Can you work these out from the model? Positions are in its coordinate system, mm. Face numbers are marked on the shaded views. A direction names the side the tool comes from. Round coordinates to 2 decimals unless told otherwise and drop trailing zeros. Order: outer loops, then holes, each group sorted by start corner. A loop starts at its lowest first (then second) coordinate and runs counter-clockwise, first axis right, second up. Notation, with made-up numbers: M 36,55 L 56,55 A26 ccw 56,75 Z; hole C -38.75,44 d2. An arc over 180 degrees is marked long. Answer as a JSON object with one key per item and string values. Group by question number.
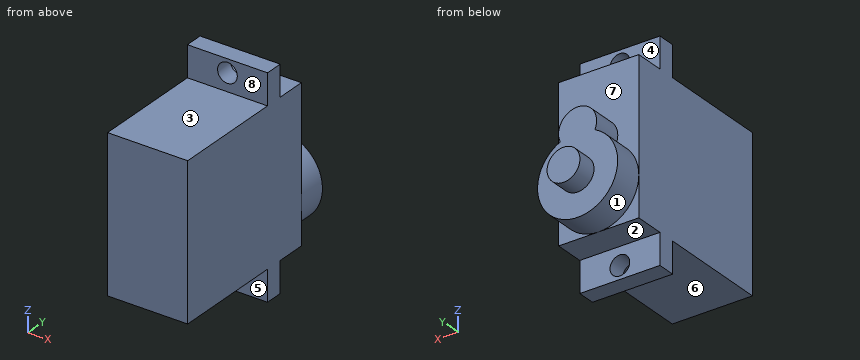
from build123d import *

# Parameters (mm, degrees)
SKETCH1_W           = 12.2
SKETCH1_H           = 23.2
BOSS_EXTRUDE3_DEPTH = 24.2
SKETCH5_W           = 12.2
SKETCH5_H           = 2.7
BOSS_EXTRUDE4_DEPTH = 4.7
CUT_EXTRUDE4_START  = -20.7
SKETCH6_R           = 1.5
CUT_EXTRUDE4_DEPTH  = 26.2
SKETCH7_R           = 2.9
SKETCH7_R_2         = 6.1
BOSS_EXTRUDE5_DEPTH = 4.5
SKETCH8_R           = 2.5
BOSS_EXTRUDE6_DEPTH = 3


with BuildPart() as part:
    # Sketch1 → Boss-Extrude3 (new body)
    with BuildSketch(Plane(origin=(0, 0, 0), x_dir=(1, 0, 0), z_dir=(0, 1, 0))):
        Rectangle(SKETCH1_W, SKETCH1_H)
    extrude(amount=BOSS_EXTRUDE3_DEPTH)

    # Sketch5 → Boss-Extrude4 (add)
    with BuildSketch(Plane.XY.offset(11.6)):
        with Locations((0, 18.35)):
            Rectangle(SKETCH5_W, SKETCH5_H)
    boss_extrude4 = extrude(amount=BOSS_EXTRUDE4_DEPTH)

    # Sketch6 → Cut-Extrude4 (cut)
    with BuildSketch(Plane(origin=(0, 19.7, 0), x_dir=(1, 0, 0), z_dir=(0, 1, 0)).offset(CUT_EXTRUDE4_START)):
        with Locations((0, -14.3)):
            Circle(SKETCH6_R)
    cut_extrude4 = extrude(amount=CUT_EXTRUDE4_DEPTH, mode=Mode.SUBTRACT)

    # Mirror3: Boss-Extrude4, Cut-Extrude4 across plane
    add(boss_extrude4.mirror(Plane.XY))
    add(cut_extrude4.mirror(Plane.XY), mode=Mode.SUBTRACT)

    # Sketch7 → Boss-Extrude5 (add)
    with BuildSketch(Plane(origin=(0, 24.2, 0), x_dir=(1, 0, 0), z_dir=(0, 1, 0))):
        with Locations((0, -1.2)):
            Circle(SKETCH7_R)
        with Locations((0, 5.5)):
            Circle(SKETCH7_R_2)
    extrude(amount=BOSS_EXTRUDE5_DEPTH)

    # Sketch8 → Boss-Extrude6 (add)
    with BuildSketch(Plane(origin=(0, 28.7, 0), x_dir=(1, 0, 0), z_dir=(0, 1, 0))):
        with Locations((0, 5.5)):
            Circle(SKETCH8_R)
    extrude(amount=BOSS_EXTRUDE6_DEPTH)


solid = part.part
Item 1: I'm going to push flat-ended pins straight in: pin 1 Ø5 at (x, z) = (0.5, -14.5) entering from -Y; pin 2 Ø5 at (x, z) = (3, 14.5) entering from +Y; pin 3 Ø1.3 at (x, y) = (-1.5, 21.5) entering from +Z. Where does each tip first touch, or does it pass through?
Item 2: On a 3-axis mill with a long thin cutter (end or side, diameter ignored), from which of +Z, -Z, +X, -X, +Y, -Y can I reach the whole of each face in a straight line? I mean the marked faces 1, 2, 3, 4 and 5. Say none if no direction works.
Item 3: Suppose I cut it at D-D, the plane x = -0.75. Write out the boundary of the cut face in (y, z).
Item 4: Suppose I cut it at A-A, the plane y = 19. Write out the boundary of the cut face in (x, z).
Item 5: If we mould it in two halves opening along Y, with no side actions, what happens to the marked faces 6, 7 and 8? For each: +Y half, -Y half, draft (parallel to the pull), parting line (faces both ways), or undercut.
Item 6: Suppose I cut it at B-B, the plane z = -14.3. Write out the boundary of the cut face in (x, y).
Item 7: I need wall thicknesses on line 1 (Z direction, x = 0, y = 17.7); line 2 (Y direction, x = 0.5, z = 4.5); line 3 (Y direction, x = -0.75, z = 1). Which ranges of each line are inside material? Lowest first, please.
Item 8: Suppose I cut it at C-C, the plane z = 1.2. Write out the boundary of the cut face in (x, y), and give its area (3 significant figures).
Computed:
{
 "1": {"pin 1": "stops at y = 17", "pin 2": "stops at y = 19.7", "pin 3": "stops at z = 11.6"},
 "2": {"face 1": "+Y", "face 2": "-Z, +X, -X, +Y", "face 3": "+Z, +X, -X, -Y", "face 4": "+Z, +X, -X, +Y", "face 5": "-Z, +X, -X, -Y"},
 "3": {"outline": "M 0,-11.6 L 17,-11.6 L 17,-13 L 19.7,-13 L 19.7,-11.6 L 24.2,-11.6 L 24.2,-11.55 L 28.7,-11.55 L 28.7,-7.88 L 31.7,-7.88 L 31.7,-3.12 L 28.7,-3.12 L 28.7,4 L 24.2,4 L 24.2,11.6 L 19.7,11.6 L 19.7,13 L 17,13 L 17,11.6 L 0,11.6 Z; M 17,-16.3 L 19.7,-16.3 L 19.7,-15.6 L 17,-15.6 Z; M 17,15.6 L 19.7,15.6 L 19.7,16.3 L 17,16.3 Z"},
 "4": {"outline": "M -6.1,-16.3 L 6.1,-16.3 L 6.1,16.3 L -6.1,16.3 Z; hole C 0,-14.3 d3; hole C 0,14.3 d3"},
 "5": {"face 6": "draft", "face 7": "+Y half", "face 8": "-Y half"},
 "6": {"outline": "M -6.1,17 L -1.5,17 L -1.5,19.7 L -6.1,19.7 Z; M 1.5,17 L 6.1,17 L 6.1,19.7 L 1.5,19.7 Z"},
 "7": {"line 1": "z = -16.3 to -15.8, -12.8 to 12.8, 15.8 to 16.3", "line 2": "y = 0 to 24.2", "line 3": "y = 0 to 28.7"},
 "8": {"outline": "M -6.1,0 L 6.1,0 L 6.1,24.2 L 2.9,24.2 L 2.9,28.7 L -2.9,28.7 L -2.9,24.2 L -6.1,24.2 Z", "area": "321 mm^2"}
}
